Geometry check sheet. Reference: drawing and pictorial views, mm from the part's lowest x, y, z. A direction names the side the tool comes from. Round coordinates to 2 decimals unless told otherwise and drop trailing zeros. Write each loop counter-clockwise with the first axis right and the second up, starting at its lowest first coordinate (ties: lowest second). Pieces come first, ordered by that corner, then holes. Notation, with made-up numbers: (-29, 5) -> (18, 5) arc R18 ccw to (18, 13) -> close; hole circle Ø8 at (26, -14.75). An arc over 180 degrees is marked (long way). Answer as a JSON object with one key per item and string values. Group by question number.
(1) Draft check along Y on the marked faces 1, 2, 3 and 4. Enter one of: released by +Y, released by -Y, zero draft, split by the parting line, or undercut.
(2) Set-up check for the marked faces 5 and 6: record each of +Z, -Z, +X, -X, +Y, -Y from which the full face is reachable in a straight line by a thin tool's end or side.
(3) Sectioned sample at C-C on y = 3.75. Record the cut outline in (x, z) (1 decimal).
(4) Sectioned sample at B-B on z = 7. Record the cut outline in (x, y).
(5) Gauge pin test, flat ends, axial feed: pin 1 Ø0.8 at (x, y) = (0.5, 20) entering from -Z; pin 2 Ø2.5 at (x, y) = (3, 13) entering from +Z; pin 3 Ø1.1 at (x, z) = (0.5, 30.5) entering from -Y. Record the tip position at first contact, or that the pin passes through.
(6) Scan lines: L1, parallel to X at y = 23, z = 25; L2, parallel to Y at x = 3.2, z = 52 (1 decimal); L3, parallel to Y at x = 4.5, z = 46 (1 decimal). Record each from-to range of solid material in increasing order. Write a range as from..to.
(7) Sectioned sample at A-A on y = 24.25. Record the cut outline in (x, z), and give its area (3 significant figures).
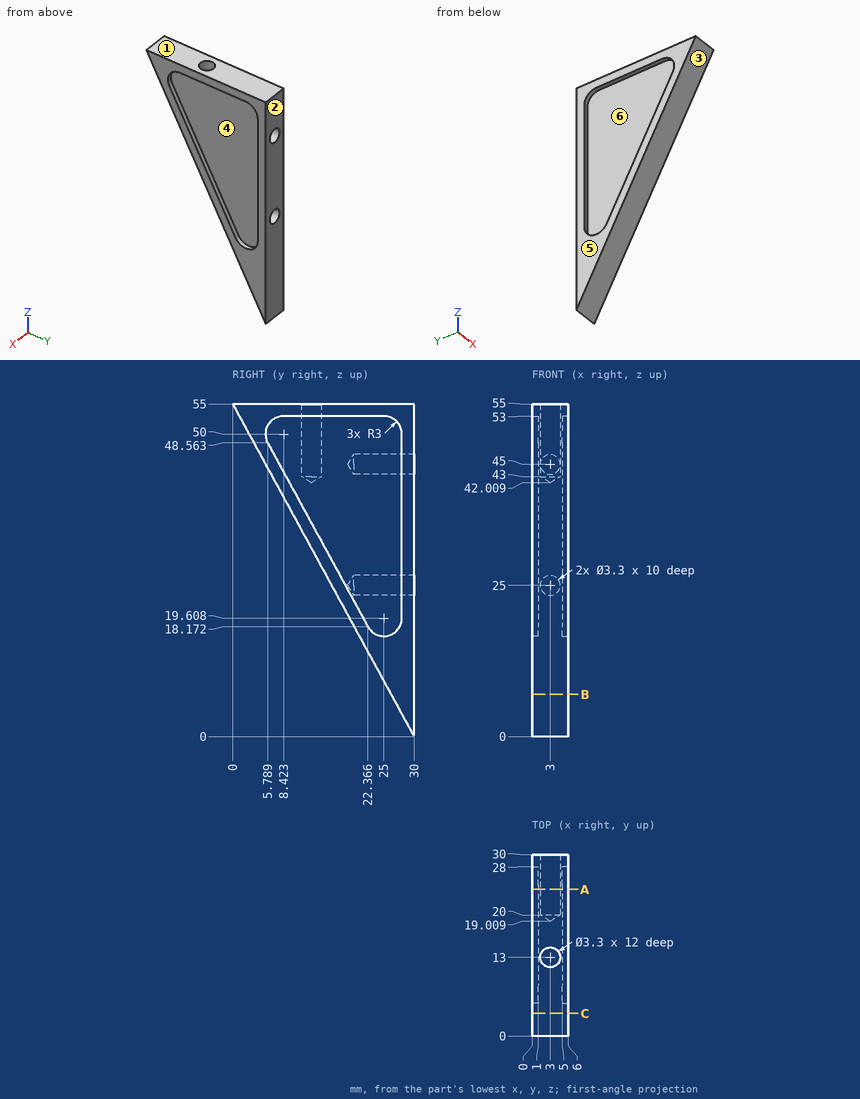
Computed values:
{
 "1": {"face 1": "zero draft", "face 2": "released by +Y", "face 3": "released by -Y", "face 4": "undercut"},
 "2": {"face 5": "+Z, -Z, -X, +Y, -Y", "face 6": "-X"},
 "3": {"outline": "(0, 48.1) -> (6, 48.1) -> (6, 55) -> (0, 55) -> close"},
 "4": {"outline": "(0, 26.18) -> (6, 26.18) -> (6, 30) -> (0, 30) -> close"},
 "5": {"pin 1": "z = 17.6", "pin 2": "z = 42.76", "pin 3": "y = 13.06"},
 "6": {"L1": "1..1.35, 4.65..5", "L2": "1.6..11.4, 14.6..30", "L3": "4.9..12.3, 13.7..30"},
 "7": {"outline": "(0, 10.54) -> (6, 10.54) -> (6, 16.7) -> (5, 16.7) -> (5, 53) -> (6, 53) -> (6, 55) -> (0, 55) -> (0, 53) -> (1, 53) -> (1, 16.7) -> (0, 16.7) -> close; hole circle Ø3.3 at (3, 25); hole circle Ø3.3 at (3, 45)", "area": "177 mm2"}
}
